For this review, use the dimensioned drawing (mm, ordinates from the lowest corner) and the shaded views. A direction names the side the tool comes from. Round coordinates to 2 decimals unless told otherwise and drop trailing zeros. Write each loop counter-clockwise with the first axis right and the second up, starting at its lowest first coordinate (ties: lowest second). Pieces come first, ordered by that corner, then holes.
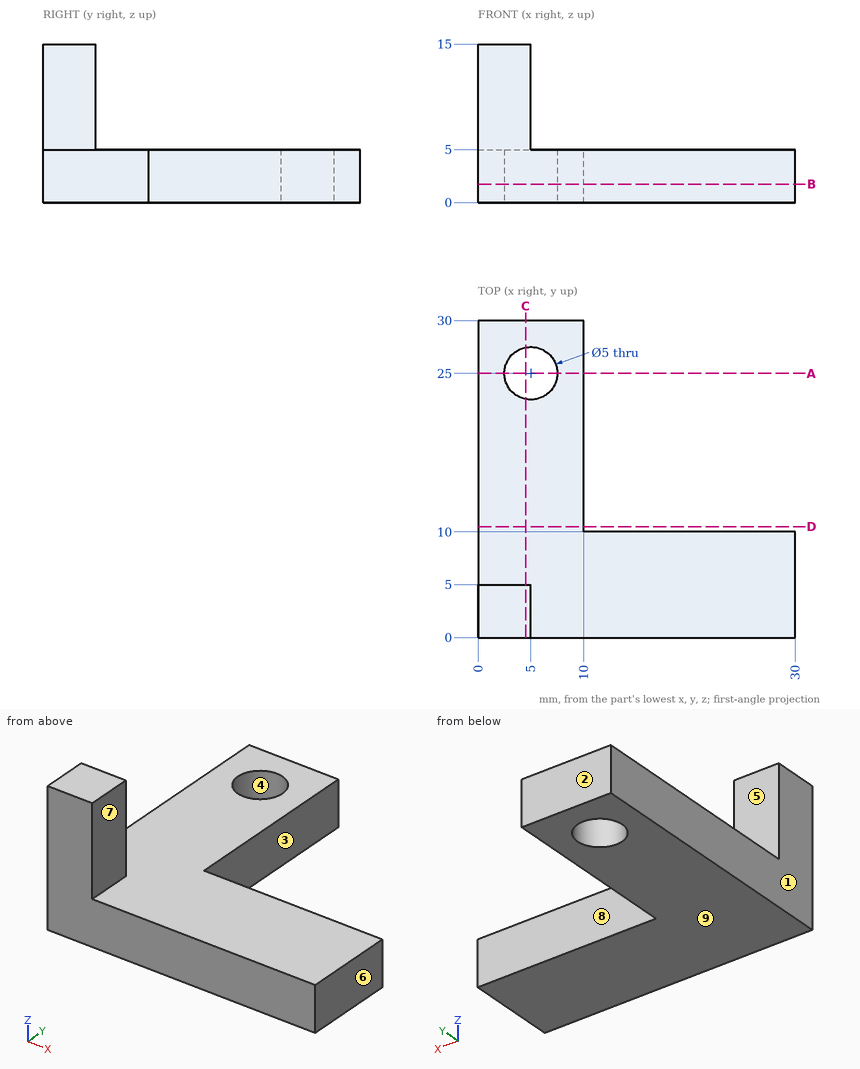
(1) For the marked faces 5, 6, 7, 8 and 9, list the 3-axis set-ups (+Z, -Z, +X, -X, +Y, -Y) from which the entire face can be reached by the end or side of a thin tool; tool diameter is ignored.
Geometry check:
face 5: +Z, +X, -X, +Y
face 6: +Z, -Z, +X, +Y, -Y
face 7: +Z, +X, +Y, -Y
face 8: +Z, -Z, +X, +Y
face 9: -Z, +X, -X, +Y, -Y
(2) For line 1 along Y through (x, z) = (5, 2.5); line 2 along Y through (x, z) = (21.75, 3.25); line 3 along Z through (x, y) = (3, 8.25), list the stretches that pass through material, from the lowest coordinate up.
Geometry check:
line 1: y = 0 to 22.5, 27.5 to 30
line 2: y = 0 to 10
line 3: z = 0 to 5
(3) For pin 1 Ø1.5 at (y, z) = (22, 2.5) entering from +X; pin 2 Ø5 at (y, z) = (7, 12) entering from -X; pin 3 Ø1.5 at (x, z) = (3, 8) entering from +Y; pin 4 Ø1.5 at (x, z) = (19.5, 3.5) entering from +Y, all flat-tipped, find the tip position at first contact; note any pin that passes through.
Geometry check:
pin 1: stops at x = 10
pin 2: stops at x = 0
pin 3: stops at y = 5
pin 4: stops at y = 10
(4) We need section C-C, the plane x = 4.5. Give the boundary of the cut face in (y, z), and give its area (3 significant figures).
Geometry check:
outline: (0, 0) - (22.55, 0) - (22.55, 5) - (5, 5) - (5, 15) - (0, 15) - close; (27.45, 0) - (30, 0) - (30, 5) - (27.45, 5) - close
area: 176 mm2
(5) We need section B-B, the plane z = 1.75. Give the boundary of the cut face in (x, y), and give its area (3 significant figures).
Geometry check:
outline: (0, 0) - (30, 0) - (30, 10) - (10, 10) - (10, 30) - (0, 30) - close; hole circle Ø5 at (5, 25)
area: 480 mm2
(6) We need section D-D, the plane y = 10.5. Give the boundary of the cut face in (x, z), and give its area (3 significant figures).
Geometry check:
outline: (0, 0) - (10, 0) - (10, 5) - (0, 5) - close
area: 50.0 mm2
(7) We need section A-A, the plane y = 25. Give the boundary of the cut face in (x, z), and give its area (3 significant figures).
Geometry check:
outline: (0, 0) - (2.5, 0) - (2.5, 5) - (0, 5) - close; (7.5, 0) - (10, 0) - (10, 5) - (7.5, 5) - close
area: 25.0 mm2
(8) Mouldability with a two-part tool opening along X and no side actions: class the marked faces 1, 2, 3 and 4 as pulls with the +X half, pulls with the -X half, needs draft (parallel to the pull), parting line crosses it, or undercut.
Geometry check:
face 1: pulls with the -X half
face 2: needs draft
face 3: pulls with the +X half
face 4: undercut
